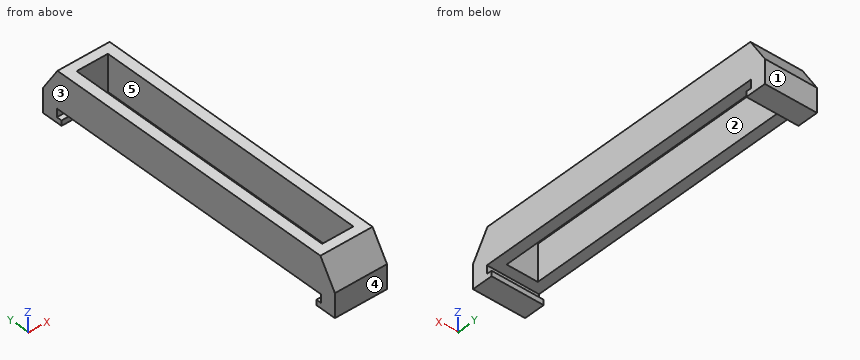
from build123d import *
from OCP.BRepFilletAPI import BRepFilletAPI_MakeChamfer

# Parameters (mm, degrees)
SZKIC3_W                    = 10
SZKIC3_H                    = 63
DODANIE_WYCI_GNI_CIE1_DEPTH = 7
WYTNIJ_WYCI_GNI_CIE1_REACH  = 66.172
SZKIC4_W                    = 6
SZKIC4_H                    = 53
SFAZOWANIE1_SIZE            = 5
SFAZOWANIE1_SIZE2           = 3.12434676
DODANIE_WYCI_GNI_CIE2_DEPTH = 10


with BuildPart() as part:
    # Szkic3 → Dodanie-wyciągnięcie1 (new body)
    with BuildSketch(Plane.XY):
        with Locations((5, 31.5)):
            Rectangle(SZKIC3_W, SZKIC3_H)
    extrude(amount=DODANIE_WYCI_GNI_CIE1_DEPTH)

    # Szkic4 → Wytnij-wyciągnięcie1 (cut, up to next)
    with BuildSketch(Plane.XY.offset(7), mode=Mode.PRIVATE) as wytnij_wyci_gni_cie1_sk1:
        with Locations((5, 31.5)):
            Rectangle(SZKIC4_W, SZKIC4_H)
    wytnij_wyci_gni_cie1_tool1 = extrude(wytnij_wyci_gni_cie1_sk1.sketch, amount=-WYTNIJ_WYCI_GNI_CIE1_REACH, mode=Mode.PRIVATE) & part.part
    add(wytnij_wyci_gni_cie1_tool1.solids().sort_by_distance((5, 31.5, 7))[0], mode=Mode.SUBTRACT)

    # Sfazowanie1: one chamfer whose edges measure the first distance from different faces: ONE call of the kernel's chamfer builder (chamfer() names one face for all edges)
    sfazowanie1_edges_1 = [part.edges().sort_by_distance(p)[0] for p in [
        (5, 63, 7),
    ]]
    sfazowanie1_side_1 = [part.faces().sort_by_distance(p)[0] for p in [
        (5, 63, 3.5),
    ]]
    sfazowanie1_edges_2 = [part.edges().sort_by_distance(p)[0] for p in [
        (5, 0, 7),
    ]]
    sfazowanie1_side_2 = [part.faces().sort_by_distance(p)[0] for p in [
        (5, 0, 3.5),
    ]]
    sfazowanie1 = BRepFilletAPI_MakeChamfer(part.part.solid().wrapped)
    for e in sfazowanie1_edges_1:
        sfazowanie1.Add(SFAZOWANIE1_SIZE, SFAZOWANIE1_SIZE2, e.wrapped, sfazowanie1_side_1[0].wrapped)  # the first distance lies on this face
    for e in sfazowanie1_edges_2:
        sfazowanie1.Add(SFAZOWANIE1_SIZE, SFAZOWANIE1_SIZE2, e.wrapped, sfazowanie1_side_2[0].wrapped)  # the first distance lies on this face
    add(Compound.cast(sfazowanie1.Shape()), mode=Mode.REPLACE)

    # Szkic6 → Dodanie-wyciągnięcie2 (add)
    with BuildSketch(Plane.ZY):
        Polygon((0, 63), (-2.6, 63), (-2.6, 59), (-1.6, 59), (-1.6, 60), (0, 60), align=None)
        Polygon((0, 0), (-2.6, 0), (-2.6, 4), (-1.6, 4), (-1.6, 3), (0, 3), align=None)
    extrude(amount=-DODANIE_WYCI_GNI_CIE2_DEPTH)


solid = part.part
Source: CAD feature listing. Evaluate the final solid. Frame: model axes, mm. Face numbers are marked on the shaded views. A direction names the side the tool comes from. Round coordinates to 2 decimals unless told otherwise and drop trailing zeros. Order: outer loops, then holes, each group sorted by start corner. A loop starts at its lowest first (then second) coordinate and runs counter-clockwise, first axis right, second up. Notation, with made-up numbers: (81, 9) - (113, 9) arc R29 cw to (113, 29) - close; hole circle Ø6 at (10, 52). An arc over 180 degrees is marked (long way). Use a Markdown table: item, result. Add a question column.
1. Line query: probe 1 along X at (y, z) = (42.5, 6.75); probe 2 along Y at (x, z) = (8.25, -0.5); probe 3 along Y at (x, z) = (3.25, 6.5). Output: solid intervals per line, ascending.
2. Section query B-B (x = 6.5). Return the cut outline in (y, z), then the cut area to 3 significant figures.
3. Section query A-A (y = 14.5). Return the cut outline in (x, z), then the cut area to 3 significant figures.
4. First-contact query: pin 1 (1.5 mm diameter, centred on x = 2.5, z = 5.5, fed in from +Y). Flat tip, straight axial feed; report the tip coordinate or a pass-through.
5. Mould query, pull axis Y, two halves, no side actions, for the marked faces 1, 2 and 3. Classes: +Y half, -Y half, draft (parallel to the pull), parting line (faces both ways), or undercut.
6. Section query D-D (x = 9.25). Return the cut outline in (y, z).
7. Section query C-C (z = 0.75). Return the cut outline in (x, y).
8. Set-up query: the marked faces 4 and 5. Return all of +Z, -Z, +X, -X, +Y, -Y with unobstructed straight access to the full face (end or side cutting, diameter ignored); none if empty.
Derived:
| question | item | result |
|---|---|---|
| 1 | probe 1 | 0 to 2, 8 to 10 |
| 1 | probe 2 | 0 to 3, 60 to 63 |
| 1 | probe 3 | 2.81 to 5, 58 to 60.19 |
| 2 | outline | (0, -2.6) - (4, -2.6) - (4, -1.6) - (3, -1.6) - (3, 0) - (5, 0) - (5, 7) - (3.12, 7) - (0, 2) - close; (58, 0) - (60, 0) - (60, -1.6) - (59, -1.6) - (59, -2.6) - (63, -2.6) - (63, 2) - (59.88, 7) - (58, 7) - close |
| 2 | area | 72.0 mm2 |
| 3 | outline | (0, 0) - (2, 0) - (2, 7) - (0, 7) - close; (8, 0) - (10, 0) - (10, 7) - (8, 7) - close |
| 3 | area | 28.0 mm2 |
| 4 | pin 1 | y = 61.28 |
| 5 | face 1 | +Y half |
| 5 | face 2 | undercut |
| 5 | face 3 | draft |
| 6 | outline | (0, -2.6) - (4, -2.6) - (4, -1.6) - (3, -1.6) - (3, 0) - (60, 0) - (60, -1.6) - (59, -1.6) - (59, -2.6) - (63, -2.6) - (63, 2) - (59.88, 7) - (3.12, 7) - (0, 2) - close |
| 7 | outline | (0, 0) - (10, 0) - (10, 63) - (0, 63) - close; hole (2, 5) - (8, 5) - (8, 58) - (2, 58) - close |
| 8 | face 4 | +Z, -Z, +X, -X, -Y |
| 8 | face 5 | +Z, -Z |
